Input: dimensioned drawing with shaded views. Units: mm. Origin: part minimum x, y, z. A direction names the side the tool comes from. Give positions to 0.01 mm unless a question says otherwise; leave off trailing zeros. Write each loop counter-clockwise with the first axis right and the second up, starting at its lowest first coordinate (ties: lowest second). Pieces come first, ordered by that corner, then holes. Notation, with made-up numbers: M 42,3.25 L 67,3.25 A32 ccw 67,33.25 Z; hole C 17,82 d6. An arc over 180 degrees is marked long. Use CSV: the item, a comma, the result in double quotes. Start each with the question number.
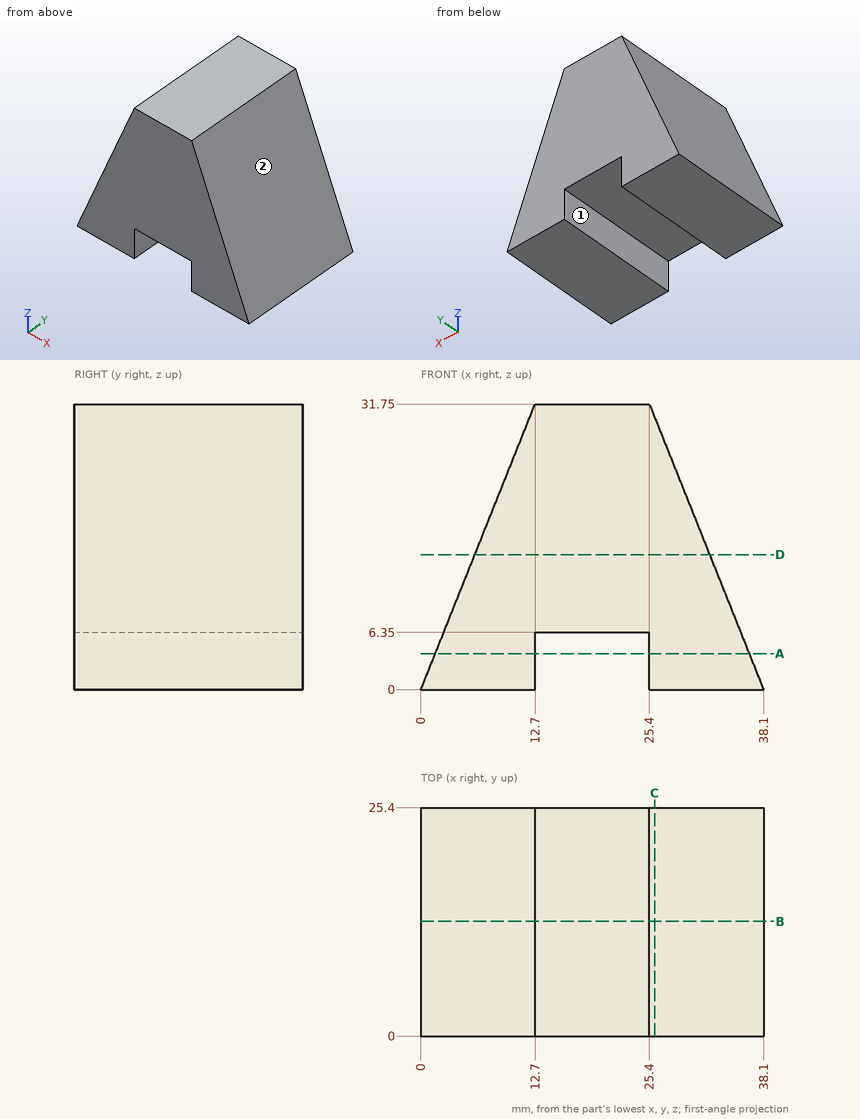
Q1. First-contact query: pin 1 Ø3 at (x, y) = (15, 6) entering from -Z; pin 2 Ø10 at (y, z) = (4, 17) entering from +X; pin 3 Ø3 at (y, z) = (10, 2) entering from -X. Flat tips, straight axial feed; report the tip coordinate or a pass-through.
Q2. Set-up query: the marked faces 1 and 2. Return all of +Z, -Z, +X, -X, +Y, -Y with unobstructed straight access to the full face (end or side cutting, diameter ignored); none if empty.
Q3. Section C-C, the plane x = 26. Return the cut outline in (y, z), and give its area (3 significant figures).
Q4. Section B-B, the plane y = 12.75. Return the cut outline in (x, z), and give its area (3 significant figures).
Q5. Section D-D, the plane z = 15. Return the cut outline in (x, y).
Q6. Section A-A, the plane z = 4. Return the cut outline in (x, y), and give its area (3 significant figures).
Q7. Material intervals for L1, parallel to Z at x = 25, y = 15; L2, parallel to X at y = 16.5, z = 2.5; L3, parallel to X at y = 15.5, z = 22, sorted ascending. Write a range as [from, to].
Check result:
1,pin 1,"stops at z = 6.35"
1,pin 2,"stops at x = 33.3"
1,pin 3,"stops at x = 0.2"
2,face 1,"-Z, +Y, -Y"
2,face 2,"+Z, +X, +Y, -Y"
3,outline,"M 0,0 L 25.4,0 L 25.4,30.25 L 0,30.25 Z"
3,area,"768 mm²"
4,outline,"M 0,0 L 12.7,0 L 12.7,6.35 L 25.4,6.35 L 25.4,0 L 38.1,0 L 25.4,31.75 L 12.7,31.75 Z"
4,area,"726 mm²"
5,outline,"M 6,0 L 32.1,0 L 32.1,25.4 L 6,25.4 Z"
6,outline,"M 1.6,0 L 12.7,0 L 12.7,25.4 L 1.6,25.4 Z; M 25.4,0 L 36.5,0 L 36.5,25.4 L 25.4,25.4 Z"
6,area,"564 mm²"
7,L1,"z = [6.35, 31.75]"
7,L2,"x = [1, 12.7], [25.4, 37.1]"
7,L3,"x = [8.8, 29.3]"
